Part model, mm, in its own coordinate system. Round coordinates to 2 decimals unless told otherwise and drop trailing zeros. Write each loop counter-clockwise with the first axis right and the second up, starting at its lowest first coordinate (ties: lowest second). Pieces come first, ordered by that corner, then holes.
```python
from build123d import *

# Parameters (mm, degrees)
SKETCH1_W           = 133
SKETCH1_H           = 58
BOSS_EXTRUDE1_DEPTH = 1
CUT_EXTRUDE1_REACH  = 74.555
FILLET1_R           = 5
CUT_EXTRUDE2_REACH  = 74.555
SKETCH3_R           = 2.6


with BuildPart() as part:
    # Sketch1 → Boss-Extrude1 (new body)
    with BuildSketch(Plane.XY):
        Rectangle(SKETCH1_W, SKETCH1_H)
    extrude(amount=BOSS_EXTRUDE1_DEPTH)

    # Sketch2 → Cut-Extrude1 (cut, up to next)
    with BuildSketch(Plane.XY, mode=Mode.PRIVATE) as cut_extrude1_sk1:
        with BuildLine():
            Line((-22.4, -18), (22.4, -18))
            ThreePointArc((22.4, -18), (22.470710678, -17.970710678), (22.5, -17.9))
            Line((22.5, -17.9), (22.5, 17.9))
            ThreePointArc((22.5, 17.9), (22.470710678, 17.970710678), (22.4, 18))
            Line((22.4, 18), (-22.4, 18))
            ThreePointArc((-22.4, 18), (-22.470710678, 17.970710678), (-22.5, 17.9))
            Line((-22.5, 17.9), (-22.5, -17.9))
            ThreePointArc((-22.5, -17.9), (-22.470710678, -17.970710678), (-22.4, -18))
        make_face()
    cut_extrude1_tool1 = extrude(cut_extrude1_sk1.sketch, amount=CUT_EXTRUDE1_REACH, mode=Mode.PRIVATE) & part.part
    add(cut_extrude1_tool1.solids().sort_by_distance((0, 0, 0))[0], mode=Mode.SUBTRACT)

    # Fillet1
    fillet1_edges = [part.edges().sort_by_distance(p)[0] for p in [
        (66.5, -29, 0.5),
        (-66.5, -29, 0.5),
        (-66.5, 29, 0.5),
        (66.5, 29, 0.5),
    ]]
    fillet(fillet1_edges, radius=FILLET1_R)

    # Sketch3 → Cut-Extrude2 (cut, up to next)
    with BuildSketch(Plane.XY, mode=Mode.PRIVATE) as cut_extrude2_sk1:
        with Locations(Location((-60, 22.5, 0), (0, 0, 180))):
            Circle(SKETCH3_R)
    cut_extrude2_tool1 = extrude(cut_extrude2_sk1.sketch, amount=CUT_EXTRUDE2_REACH, mode=Mode.PRIVATE) & part.part
    # Sketch3 → Cut-Extrude2 (cut, up to next)
    with BuildSketch(Plane.XY, mode=Mode.PRIVATE) as cut_extrude2_sk2:
        with Locations(Location((60, 22.5, 0), (0, 0, 180))):
            Circle(SKETCH3_R)
    cut_extrude2_tool2 = extrude(cut_extrude2_sk2.sketch, amount=CUT_EXTRUDE2_REACH, mode=Mode.PRIVATE) & part.part
    # Sketch3 → Cut-Extrude2 (cut, up to next)
    with BuildSketch(Plane.XY, mode=Mode.PRIVATE) as cut_extrude2_sk3:
        with Locations(Location((60, -22.5, 0), (0, 0, 180))):
            Circle(SKETCH3_R)
    cut_extrude2_tool3 = extrude(cut_extrude2_sk3.sketch, amount=CUT_EXTRUDE2_REACH, mode=Mode.PRIVATE) & part.part
    # Sketch3 → Cut-Extrude2 (cut, up to next)
    with BuildSketch(Plane.XY, mode=Mode.PRIVATE) as cut_extrude2_sk4:
        with Locations(Location((-60, -22.5, 0), (0, 0, 180))):
            Circle(SKETCH3_R)
    cut_extrude2_tool4 = extrude(cut_extrude2_sk4.sketch, amount=CUT_EXTRUDE2_REACH, mode=Mode.PRIVATE) & part.part
    add(cut_extrude2_tool1.solids().sort_by_distance((-60, 22.5, 0))[0], mode=Mode.SUBTRACT)
    add(cut_extrude2_tool2.solids().sort_by_distance((60, 22.5, 0))[0], mode=Mode.SUBTRACT)
    add(cut_extrude2_tool3.solids().sort_by_distance((60, -22.5, 0))[0], mode=Mode.SUBTRACT)
    add(cut_extrude2_tool4.solids().sort_by_distance((-60, -22.5, 0))[0], mode=Mode.SUBTRACT)


solid = part.part
```
Q1. Mould opens along Y. For faces 1 (the flat face through (-1, 20, 0)), 2 (the cylindrical face through (-57.4, 22.4, 0.5)), 3 (the cylindrical face through (65, -27.57, 0.51)), 4 (the cylindrical face through (62.6, -22.6, 0.5)) say: +Y half, -Y half, draft (parallel to the pull), parting line (faces both ways), or undercut.
Values follow:
face 1: draft
face 2: undercut
face 3: -Y half
face 4: undercut
Q2. Cut at A-A on z = 0.45. Write the cut outline in (x, y), plus the area to 3 significant figures.
Values follow:
outline: (-66.5, -24) arc R5 ccw to (-61.5, -29) - (61.5, -29) arc R5 ccw to (66.5, -24) - (66.5, 24) arc R5 ccw to (61.5, 29) - (-61.5, 29) arc R5 ccw to (-66.5, 24) - close; hole circle Ø5.2 at (-60, -22.5); hole circle Ø5.2 at (-60, 22.5); hole (-22.5, -17.9) arc R0.1 ccw to (-22.4, -18) - (22.4, -18) arc R0.1 ccw to (22.5, -17.9) - (22.5, 17.9) arc R0.1 ccw to (22.4, 18) - (-22.4, 18) arc R0.1 ccw to (-22.5, 17.9) - close; hole circle Ø5.2 at (60, -22.5); hole circle Ø5.2 at (60, 22.5)
area: 5,990 mm2
Q3. Drop a flat-ended pin along its axis: pin 1 (4 mm diameter, centred on x = 60, y = -22.5, fed in from -Z). Give the stop position or say it passes through.
Values follow:
pin 1: passes through
Q4. Wall check: L1, parallel to Y at x = -60, z = 0.7; L2, parallel to X at y = 22.5, z = 0.7; L3, parallel to X at y = 6.5, z = 0.7. Give the ranges that are in metal, low to high.
Values follow:
L1: y = -29 to -25.1, -19.9 to 19.9, 25.1 to 29
L2: x = -66.5 to -62.6, -57.4 to 57.4, 62.6 to 66.5
L3: x = -66.5 to -22.5, 22.5 to 66.5
Q5. Cut at C-C on y = -22.5. Write the cut outline in (x, z), plus the area to 3 significant figures.
Values follow:
outline: (-66.5, 0) - (-62.6, 0) - (-62.6, 1) - (-66.5, 1) - close; (-57.4, 0) - (57.4, 0) - (57.4, 1) - (-57.4, 1) - close; (62.6, 0) - (66.5, 0) - (66.5, 1) - (62.6, 1) - close
area: 123 mm2
Q6. Cut at D-D on x = -60. Write the cut outline in (y, z).
Values follow:
outline: (-29, 0) - (-25.1, 0) - (-25.1, 1) - (-29, 1) - close; (-19.9, 0) - (19.9, 0) - (19.9, 1) - (-19.9, 1) - close; (25.1, 0) - (29, 0) - (29, 1) - (25.1, 1) - close
Q7. Cut at B-B on x = -11.5. Write the cut outline in (y, z), plus the area to 3 significant figures.
Values follow:
outline: (-29, 0) - (-18, 0) - (-18, 1) - (-29, 1) - close; (18, 0) - (29, 0) - (29, 1) - (18, 1) - close
area: 22.0 mm2
